from build123d import *

# Parameters (mm, degrees)
F0_R     = 15.875
F1_DEPTH = 1.5875
F2_R     = 6.35
F3_DEPTH = 19.05
F5_DEPTH = 20.6385


with BuildPart() as f1:
    # F0 (on Top) → F1 (new body)
    with BuildSketch(Plane.XY):
        Circle(F0_R)
    extrude(amount=F1_DEPTH)

    # F2 (on face) → F3 (join)
    with BuildSketch(Plane.XY.offset(1.5875)):
        Circle(F2_R)
    extrude(amount=F3_DEPTH)

    # F4 (on face) → F5 (cut, through all)
    with BuildSketch(Plane.XY.offset(20.6375)):
        with BuildLine():
            Line((15.795426, 1.5875), (4.490128, 1.5875))
            ThreePointArc((4.490128, 1.5875), (-4.7625, 0), (4.490128, -1.5875))
            Line((4.490128, -1.5875), (15.795426, -1.5875))
            ThreePointArc((15.795426, -1.5875), (15.875, 0), (15.795426, 1.5875))
        make_face()
    extrude(amount=-F5_DEPTH, mode=Mode.SUBTRACT)


solid = f1.part
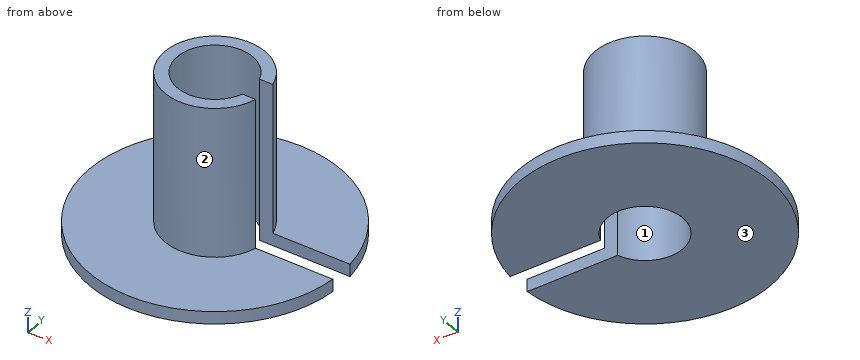
Design review of the part built by this model. Coordinates are the model's own, in mm. Face numbers are marked on the shaded views. Give positions to 0.01 mm unless a question says otherwise; leave off trailing zeros. Loops run counter-clockwise (first coordinate to the right, second up) from the corner with the lowest first, then second, coordinate; pieces in that order, holes last. Notation, with made-up numbers: (13.25, 19) - (65.25, 19) arc R25 ccw to (65.25, 57) - close; hole circle Ø8 at (85.25, 60). An arc over 180 degrees is marked (long way). Write item = value, one per line.
1) Take a section at D-D on x = 7. State the section outline as (y, z) points, and give its area (3 significant figures).
Result sheet:
outline = (-14.25, 0) - (-1.59, 0) - (-1.59, 1.59) - (-14.25, 1.59) - close; (1.59, 0) - (14.25, 0) - (14.25, 1.59) - (1.59, 1.59) - close
area = 40.2 mm2
2) To check wall thickness, follow line 1 (Y direction, x = 0, z = 11.5); line 2 (X direction, y = 0, z = 7.25); line 3 (Z direction, x = -1.5, y = 10.5). State the ranges of each line that lie inside material, in increasing order.
Result sheet:
line_1 = -6.35 to -4.76, 4.76 to 6.35
line_2 = -6.35 to -4.76
line_3 = 0 to 1.59
3) Draft analysis for pull direction X (two halves, no side actions). For the marked faces 1, 2 and 3, state which applies: +X half, -X half, draft (parallel to the pull), parting line (faces both ways), or undercut.
Result sheet:
face_1 = undercut
face_2 = parting line
face_3 = draft
4) Take a section at B-B on y = 4. State the section outline as (x, z) points, and give its area (3 significant figures).
Result sheet:
outline = (-15.36, 0) - (-2.58, 0) - (-2.58, 20.64) - (-4.93, 20.64) - (-4.93, 1.59) - (-15.36, 1.59) - close; (2.58, 0) - (15.36, 0) - (15.36, 1.59) - (4.93, 1.59) - (4.93, 20.64) - (2.58, 20.64) - close
area = 130 mm2
5) Clearance check with flat-ended pins moving along their axes: pin 1 Ø1.5 at (x, y) = (3, 11.5) entering from +Z; pin 2 Ø12 at (y, z) = (1.5, 18) entering from +X. State where each tip first meets the part, or that it passes through.
Result sheet:
pin_1 = 1.59
pin_2 = 6.15
